Input: part model. Units: mm. Frame: model coordinates. A direction names the side the tool comes from. Round coordinates to 2 decimals unless told otherwise and drop trailing zeros. Loops run counter-clockwise (first coordinate to the right, second up) from the corner with the lowest first, then second, coordinate; pieces in that order, holes last. Notation, with made-up numbers: (-5.5, 6.25) -> (46.5, 6.25) arc R27 cw to (46.5, 42.25) -> close; hole circle Ø4 at (51, 26.25). An arc over 180 degrees is marked (long way). Answer as a JSON object with one key per item and string values. Group by question number.
Item 1: Section query C-C on x = 49. Return loops of the section in (y, z), and give its area (3 significant figures).
Item 2: Section query A-A on y = 43.9. Return loops of the section in (x, z).
Item 3: Section query D-D on z = -14.5. Return loops of the section in (x, y).
Item 4: Set-up query: faces 4 (the flat face through (94, 35, 1)), 5 (the flat face through (69, 6.35, 2)), 6 (the cylindrical face through (49.208, 65.586, -29.535)). Return all of +Z, -Z, +X, -X, +Y, -Y with unobstructed straight access to the full face (end or side cutting, diameter ignored); none if empty.
Item 5: Draft query along X for faces 1 (the flat face through (54.008, 4, 2)), 2 (the flat face through (50.3, 4.7, -32)), 3 (the cylindrical face through (46, 6, -16)). Return one class per face: released by +X, released by -X, zero draft, split by the parting line, or undercut.
Item 6: Pin query (flat end, axial travel): pin 1 (3.5 mm diameter, centred on y = 64.5, z = 1, fed in from -X); pin 2 (8 mm diameter, centred on x = 75.5, y = 24.5, fed in from -Z); pin 3 (10 mm diameter, centred on x = 51, z = -15.5, fed in from +Y); pin 4 (1.6 mm diameter, centred on x = 5.5, y = 64.5, fed in from -Z). Return the tip coordinate at first contact, or that it passes through.
Item 7: Section query B-B on x = 59.5. Return loops of the section in (y, z).
Item 8: Material intervals for line 1 (Y direction, x = 49, z = -29.8); line 2 (Y direction, x = 6, z = -28); line 3 (Z direction, x = 44.5, y = 25), sorted ascending. Write a range as [from, to].
from build123d import *

# Parameters (mm, degrees)
SKETCH1_W           = 94
SKETCH1_H           = 70
BOSS_EXTRUDE2_DEPTH = 3
SKETCH3_R           = 3
BOSS_EXTRUDE5_DEPTH = 35
SKETCH7_R           = 1.602627629
CUT_EXTRUDE1_DEPTH  = 5
SKETCH8_R           = 1.6
CUT_EXTRUDE2_DEPTH  = 5
SKETCH9_R           = 1.6
CUT_EXTRUDE3_DEPTH  = 5
SKETCH10_W          = 30
SKETCH10_H          = 4
SKETCH10_R          = 1.6
SKETCH10_R_2        = 1.619244763
CUT_EXTRUDE5_DEPTH  = 5


with BuildPart() as part:
    # Sketch1 → Boss-Extrude2 (new body)
    with BuildSketch(Plane.XY):
        with Locations((47, 35)):
            Rectangle(SKETCH1_W, SKETCH1_H)
    extrude(amount=BOSS_EXTRUDE2_DEPTH)

    # Sketch3 → Boss-Extrude5 (add)
    with BuildSketch(Plane.XY.offset(3)):
        with Locations((49, 6)):
            Circle(SKETCH3_R)
        with Locations((49, 64)):
            Circle(SKETCH3_R)
        with Locations((6, 64)):
            Circle(SKETCH3_R)
    extrude(amount=-BOSS_EXTRUDE5_DEPTH)

    # Sketch7 → Cut-Extrude1 (cut)
    with BuildSketch(Plane(origin=(0, 0, -32), x_dir=(-1, 0, 0), z_dir=(0, 0, -1))):
        with Locations((-49, 6)):
            Circle(SKETCH7_R)
    extrude(amount=-CUT_EXTRUDE1_DEPTH, mode=Mode.SUBTRACT)

    # Sketch8 → Cut-Extrude2 (cut)
    with BuildSketch(Plane(origin=(0, 0, -32), x_dir=(-1, 0, 0), z_dir=(0, 0, -1))):
        with Locations((-6, 64)):
            Circle(SKETCH8_R)
    extrude(amount=-CUT_EXTRUDE2_DEPTH, mode=Mode.SUBTRACT)

    # Sketch9 → Cut-Extrude3 (cut)
    with BuildSketch(Plane(origin=(0, 0, -32), x_dir=(-1, 0, 0), z_dir=(0, 0, -1))):
        with Locations((-49, 64)):
            Circle(SKETCH9_R)
    extrude(amount=-CUT_EXTRUDE3_DEPTH, mode=Mode.SUBTRACT)

    # Sketch10 → Cut-Extrude5 (cut)
    with BuildSketch(Plane.XY.offset(3)):
        with Locations((69.008203537, 65.665805626)):
            Rectangle(SKETCH10_W, SKETCH10_H)
        with Locations((69.008203537, 4.35)):
            Rectangle(SKETCH10_W, SKETCH10_H)
        with Locations((29.408203537, 10.85)):
            Circle(SKETCH10_R)
        with Locations((81.508203537, 15.998164517)):
            Circle(SKETCH10_R)
        with Locations((81.508203537, 43.9)):
            Circle(SKETCH10_R)
        with Locations((30.708203537, 59.1)):
            Circle(SKETCH10_R_2)
    extrude(amount=-CUT_EXTRUDE5_DEPTH, mode=Mode.SUBTRACT)


solid = part.part
Solved:
{
 "1": {"outline": "(0, 0) -> (3, 0) -> (3, -32) -> (4.4, -32) -> (4.4, -27) -> (7.6, -27) -> (7.6, -32) -> (9, -32) -> (9, 0) -> (61, 0) -> (61, -32) -> (62.4, -32) -> (62.4, -27) -> (65.6, -27) -> (65.6, -32) -> (67, -32) -> (67, 0) -> (70, 0) -> (70, 3) -> (0, 3) -> close", "area": "562 mm²"},
 "2": {"outline": "(0, 0) -> (79.91, 0) -> (79.91, 3) -> (0, 3) -> close; (83.11, 0) -> (94, 0) -> (94, 3) -> (83.11, 3) -> close"},
 "3": {"outline": "circle Ø6 at (6, 64); circle Ø6 at (49, 6); circle Ø6 at (49, 64)"},
 "4": {"face 4": "+Z, -Z, +X, +Y, -Y", "face 5": "+Z, -Z", "face 6": "-Z"},
 "5": {"face 1": "undercut", "face 2": "zero draft", "face 3": "split by the parting line"},
 "6": {"pin 1": "x = 0", "pin 2": "z = 0", "pin 3": "y = 67", "pin 4": "z = -27"},
 "7": {"outline": "(0, 0) -> (2.35, 0) -> (2.35, 3) -> (0, 3) -> close; (6.35, 0) -> (63.67, 0) -> (63.67, 3) -> (6.35, 3) -> close; (67.67, 0) -> (70, 0) -> (70, 3) -> (67.67, 3) -> close"},
 "8": {"line 1": "[3, 4.4], [7.6, 9], [61, 62.4], [65.6, 67]", "line 2": "[61, 62.4], [65.6, 67]", "line 3": "[0, 3]"}
}
